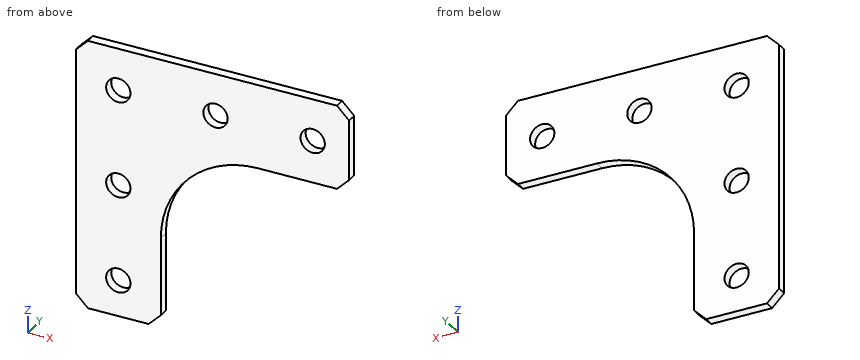
Autodesk Inventor part; units mm, degrees
ref_plane "YZ Plane" through (0, 0, 0) normal (1, 0, 0) x (0, 1, 0)
ref_plane "XZ Plane" through (0, 0, 0) normal (0, 1, 0) x (-1, 0, 0)
ref_plane "XY Plane" through (0, 0, 0) normal (0, 0, 1) x (1, 0, 0)
sketch "Sketch1" plane through (0, 0, 0) normal (0, 1, 0) x (-1, 0, 0)
  line L0 (-3.175, 0) -> (-19.05, 0)
  line L1 (-71.4375, 52.3875) -> (-71.4375, 68.2625)
  line L2 (-68.2625, 71.4375) -> (-3.175, 71.4375)
  line L3 (0, 68.2625) -> (0, 3.175)
  line L4 (-3.175, 0) -> (0, 3.175)
  line L5 (0, 68.2625) -> (-3.175, 71.4375)
  line L6 (-68.2625, 71.4375) -> (-71.4375, 68.2625)
  line L7 (-22.225, 3.175) -> (-22.225, 23.8125)
  line L8 (-47.625, 49.2125) -> (-68.2625, 49.2125)
  arc A0 (-22.225, 23.8125) -> (-47.625, 49.2125) centre (-47.625, 23.8125) ccw
  line L9 (-22.225, 3.175) -> (-19.05, 0)
  line L10 (-71.4375, 52.3875) -> (-68.2625, 49.2125)
  point P0 (0, 0)
  point P1 (-71.4375, 71.4375)
  point P2 (0, 71.4375)
  point P3 (-22.225, 49.2125)
  point P4 (-22.225, 0)
  point P5 (-71.4375, 49.2125)
  dimension "d0" = 71.4375
  dimension "d2" = 3.175
  dimension "d3" = 3.175
  dimension "d4" = 3.175
  dimension "d5" = 3.175
  dimension "d6" = 3.175
  dimension "d7" = 3.175
  dimension "d11" = 3.175
  dimension "d12" = 3.175
  dimension "d13" = 3.175
  dimension "d14" = 3.175
  dimension "d32" = 15.875
  dimension "d35" = 15.875
  dimension "d37" = 71.4375
  dimension "d38" = 25.4
  dimension "d39" = 47.625
  dimension "d40" = 47.625
extrude "Extrusion1" add sketch "Sketch1" along normal blind 2.54
hole "Hole1" at (11.1125, 2.54, 60.325) direction (0, -1, 0) diameter 6.35 end through all
pattern_linear "Rectangular Pattern1" count 3 spacing 25.4 along (0, 0, -1) of "Hole1"
pattern_linear "Rectangular Pattern2" count 3 spacing 25.4 along (1, 0, 0) of "Hole1"
equation "\"d35\" = d32"
equation "\"d37\" = d0"
equation "\"d40\" = d39"
equation "\"BendRadius\" = Thickness"
equation "\"BendReliefWidth\" = Thickness"
equation "\"BendReliefDepth\" = 0.5 * Thickness"
equation "\"CornerReliefSize\" = 4 * Thickness"
equation "\"MinimumRemnant\" = 2 * Thickness"
equation "\"TransitionRadius\" = BendRadius"
equation "\"JacobiRadiusSize\" = Thickness"
equation "\"GapSize\" = Thickness"
properties part number "3x3 Gusset"
Verification items for the finished model (mm, model axes). Give positions to 0.01 mm unless a question says otherwise; leave off trailing zeros. Loops run counter-clockwise (first coordinate to the right, second up) from the corner with the lowest first, then second, coordinate; pieces in that order, holes last.
1) Sectioned sample at C-C, the plane x = 50. Enter the section's corners in (y, z).
2) Sectioned sample at A-A, the plane x = 38.5. Enter the section's corners in (y, z).
3) Sectioned sample at D-D, the plane z = 42.5. Enter the section's corners in (x, y), then the cut area to 3 significant figures.
4) Thickness scan on line 1 along X through (y, z) = (2.1, 59.5); line 2 along Z through (x, y) = (14, 0.35); line 3 along Z through (x, y) = (11.5, 0.25). Record the ranges inside material, lowest first.
5) Depth check by flat-ended pin: pin 1 Ø5 at (x, z) = (11.11, 9.52) entering from -Y (3 decimals); pin 2 Ø10 at (x, z) = (11.11, 60.32) entering from +Y; pin 3 Ø0.8 at (y, z) = (2, 14) entering from +X (3 decimals). Enter the tip coordinate at first touch or a pass-through.
6) Sectioned sample at B-B, the plane y = 0.6. Count the separate pieces of the cut face and the enclosed holes in it, then the cut area to 3 significant figures.
Answers:
1. outline: (0, 49.21) - (2.54, 49.21) - (2.54, 71.44) - (0, 71.44) - close
2. outline: (0, 47.52) - (2.54, 47.52) - (2.54, 57.85) - (0, 57.85) - close; (0, 62.8) - (2.54, 62.8) - (2.54, 71.44) - (0, 71.44) - close
3. outline: (0, 0) - (30.42, 0) - (30.42, 2.54) - (0, 2.54) - close
3. area: 77.3 mm2
4. line 1: x = 0 to 8.05, 14.18 to 33.45, 39.58 to 58.85, 64.98 to 71.44
4. line 2: z = 0 to 8.2, 10.85 to 33.6, 36.25 to 59, 61.65 to 71.44
4. line 3: z = 0 to 6.37, 12.68 to 31.77, 38.08 to 57.17, 63.48 to 71.44
5. pin 1: passes through
5. pin 2: stops at y = 2.54
5. pin 3: stops at x = 22.225
6. separate pieces: 1
6. enclosed holes: 5
6. area: 2,640 mm2
